Design review of the part built by this model. Coordinates are the model's own, in mm. Face numbers are marked on the shaded views. A direction names the side the tool comes from. Round coordinates to 2 decimals unless told otherwise and drop trailing zeros. Write each loop counter-clockwise with the first axis right and the second up, starting at its lowest first coordinate (ties: lowest second). Pieces come first, ordered by that corner, then holes. Notation, with made-up numbers: (13, 15) -> (57, 15) arc R12 cw to (57, 37) -> close; hole circle Ø11 at (82.5, -10.75). An arc over 180 degrees is marked (long way). One line per question, with ' | ' between items. Start each with the question number.
1) Consider section B-B (y = 4.75). Give the boundary of the cut face in (x, z) (3 decimals), then the cut area to 3 significant figures.
2) Consider section D-D (z = -1). Give the boundary of the cut face in (x, y) (3 decimals).
3) Insertion check: pin 1 Ø3 at (y, z) = (12, -6.5) entering from +X. The pin has a flat end and moves straight along its axis. Give the tip position at first contact, or say it passes through.
4) Consider section C-C (y = 6.75). Give the boundary of the cut face in (x, z) (3 decimals).
5) For the marked faces 1 and 2, list the 3-axis set-ups (+Z, -Z, +X, -X, +Y, -Y) from which the entire face can be reached by the end or side of a thin tool; tool diameter is ignored.
6) Consider section A-A (z = 8). Give the boundary of the cut face in (x, y) (3 decimals).
7) For probe 1 along X at (y, z) = (7.25, -10) (3 decimals); probe 2 along Y at (x, z) = (-9, 10.25); probe 3 along Z at (x, y) = (-1, 2.25), list the stretches that pass through material, from the lowest coordinate up.
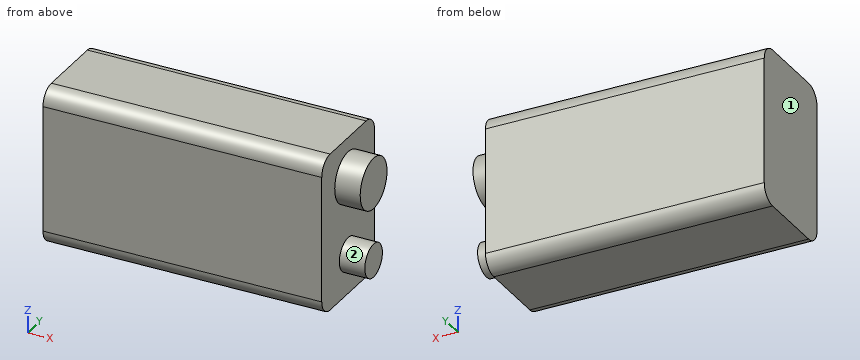
```python
from build123d import *

# Parameters (mm, degrees)
SKETCH1_W           = 44.45
SKETCH1_H           = 25.146
BOSS_EXTRUDE1_DEPTH = 16.002
FILLET1_R           = 2.54
SKETCH2_R           = 4.064
SKETCH2_R_2         = 2.667
BOSS_EXTRUDE2_DEPTH = 4.064


with BuildPart() as part:
    # Sketch1 → Boss-Extrude1 (new body)
    with BuildSketch(Plane(origin=(0, 0, 0), x_dir=(1, 0, 0), z_dir=(0, 1, 0))):
        Rectangle(SKETCH1_W, SKETCH1_H)
    extrude(amount=BOSS_EXTRUDE1_DEPTH)

    # Fillet1
    fillet1_edges = [part.edges().sort_by_distance(p)[0] for p in [
        (0, 16.002, 12.573),
        (0, 0, 12.573),
        (0, 0, -12.573),
        (0, 16.002, -12.573),
    ]]
    fillet(fillet1_edges, radius=FILLET1_R)

    # Sketch2 → Boss-Extrude2 (add)
    with BuildSketch(Plane(origin=(22.225, 0, 0), x_dir=(0, 0, -1), z_dir=(1, 0, 0))):
        with Locations(Location((-6.223, 8.001, 0), (0, 0, 180))):
            Circle(SKETCH2_R)
        with Locations(Location((6.223, 8.001, 0), (0, 0, 180))):
            Circle(SKETCH2_R_2)
    extrude(amount=BOSS_EXTRUDE2_DEPTH)


solid = part.part
```
From the geometry:
1) outline: (-22.225, -12.573) -> (22.225, -12.573) -> (22.225, 3.784) -> (26.289, 3.784) -> (26.289, 8.662) -> (22.225, 8.662) -> (22.225, 12.573) -> (-22.225, 12.573) -> close | area: 1,140 mm2
2) outline: (-22.225, 0) -> (22.225, 0) -> (22.225, 16.002) -> (-22.225, 16.002) -> close
3) pin 1: stops at x = 26.29
4) outline: (-22.225, -12.573) -> (22.225, -12.573) -> (22.225, -8.578) -> (26.289, -8.578) -> (26.289, -3.868) -> (22.225, -3.868) -> (22.225, 2.356) -> (26.289, 2.356) -> (26.289, 10.09) -> (22.225, 10.09) -> (22.225, 12.573) -> (-22.225, 12.573) -> close
5) face 1: +Z, -Z, -X, +Y, -Y | face 2: +X
6) outline: (-22.225, 0) -> (22.225, 0) -> (22.225, 4.346) -> (26.289, 4.346) -> (26.289, 11.656) -> (22.225, 11.656) -> (22.225, 16.002) -> (-22.225, 16.002) -> close
7) probe 1: x = -22.225 to 22.225 | probe 2: y = 0.01 to 15.99 | probe 3: z = -12.56 to 12.56
